from build123d import *

# Parameters (mm, degrees)
F1_DEPTH    = 30
F2_T1_DEPTH = 30
F2_T3_DEPTH = 35


# Not quite as in the source:
# - a fillet or chamfer that OpenCascade refuses, or shapes differently, is made with other operations: its cross-section is extruded or revolved along the edge and cut away or added
# - ends of sketch curves that miss each other by under 0.0002 mm in the source are joined


with BuildPart() as f1:
    # F0 (on Top) → F1 (new body)
    with BuildSketch(Plane.XY):
        with BuildLine():
            ThreePointArc((0.0108101467, 3.9999853926), (3.7311619501, 1.441676282), (2.6975556514, -2.9535052916))
            Line((2.6975556514, -2.9535052916), (3.5790398152, -3.7723300494))
            ThreePointArc((3.5790398152, -3.7723300494), (4.7376169007, -2.1435918693), (5.1962235425, -0.1981436252))
            ThreePointArc((5.1962235425, -0.1981436252), (5.1972192437, -0.0990548017), (5.2, 0))
            ThreePointArc((5.2, 0), (4.6973944029, 2.2303555374), (3.2867362218, 4.0295613915))
            Line((3.2867362218, 4.0295613915), (0.0108101467, 3.9999853926))
        make_face()
        with BuildLine():
            ThreePointArc((-2.6975556514, -2.9535052916), (-3.7272521414, 1.4517546193), (0.0108101467, 3.9999853926))
            Line((0.0108101467, 3.9999853926), (3.2867362218, 4.0295613915))
            ThreePointArc((3.2867362218, 4.0295613915), (1.7444599113, 4.8986589612), (0, 5.2))
            ThreePointArc((0, 5.2), (-4.8299128489, 1.9266400472), (-3.5790398152, -3.7723300494))
            Line((-3.5790398152, -3.7723300494), (-2.6975556514, -2.9535052916))
        make_face()
        with BuildLine():
            ThreePointArc((0, 5.2), (1.7444599113, 4.8986589612), (3.2867362218, 4.0295613915))
            Line((3.2867362218, 4.0295613915), (7.2283371129, 4.065071131))
            ThreePointArc((7.2283371129, 4.065071131), (8.8329374117, 4.9709020374), (10.646673336, 5.2959154939))
            Line((10.646673336, 5.2959154939), (0, 5.2))
        make_face()
        with BuildLine():
            ThreePointArc((5.2, 0), (5.1972192437, -0.0990548017), (5.1962235425, -0.1981436252))
            ThreePointArc((5.1962235425, -0.1981436252), (5.1990557999, -0.099089805), (5.2, 0))
        make_face()
        with BuildLine():
            ThreePointArc((5.2, 0), (5.1990557999, -0.099089805), (5.1962235425, -0.1981436252))
            ThreePointArc((5.1962235425, -0.1981436252), (5.5915030666, -2.2512643656), (6.7244861035, -4.0085065559))
            Line((6.7244861035, -4.0085065559), (7.5779271506, -3.1646460444))
            ThreePointArc((7.5779271506, -3.1646460444), (6.7375812297, 1.4751784497), (10.6574836162, 4.0959641875))
            Line((10.6574836162, 4.0959641875), (7.2283371129, 4.065071131))
            ThreePointArc((7.2283371129, 4.065071131), (5.7748395568, 2.2517463212), (5.2, 0))
        make_face()
        with BuildLine():
            ThreePointArc((10.646673336, 5.2959154939), (8.8329374117, 4.9709020374), (7.2283371129, 4.065071131))
            Line((7.2283371129, 4.065071131), (10.6574836162, 4.0959641875))
            Line((10.6574836162, 4.0959641875), (14.0866300839, 4.1268572436))
            ThreePointArc((14.0866300839, 4.1268572436), (12.4659704087, 5.0036318817), (10.646673336, 5.2959154939))
        make_face()
        with BuildLine():
            Line((16.1859897918, 5.345818995), (10.646673336, 5.2959154939))
            ThreePointArc((10.646673336, 5.2959154939), (12.4659704087, 5.0036318817), (14.0866300839, 4.1268572436))
            Line((14.0866300839, 4.1268572436), (17.6967392423, 4.1593805861))
            Line((17.6967392423, 4.1593805861), (17.6859289245, 5.3593318922))
            Line((17.6859289245, 5.3593318922), (16.1859897918, 5.345818995))
        make_face()
        with BuildLine():
            Line((14.0866300839, 4.1268572436), (10.6574836162, 4.0959641875))
            ThreePointArc((10.6574836162, 4.0959641875), (14.6395734892, 1.510772092), (13.8145139904, -3.1646460444))
            Line((13.8145139904, -3.1646460444), (14.6679550375, -4.0085065559))
            ThreePointArc((14.6679550375, -4.0085065559), (16.1822325131, 0.1881501089), (14.0866300839, 4.1268572436))
        make_face()
        Polygon((16.1634682964, 7.8457175493), (16.1859897918, 5.345818995), (17.6859289245, 5.3593318922), (17.6634074291, 7.8592304466), align=None)
        Polygon((-0.0225214954, 7.6998985544), (16.1634682964, 7.8457175493), (17.6634074291, 7.8592304466), (17.6498945318, 9.3591695792), (-0.0360343926, 9.199837687), (-4.7136558579, 9.1576971649), (-4.7001429606, 7.6577580323), align=None)
    extrude(amount=F1_DEPTH)

    # F2: fillet of radius 1 on 6 edges, made by hand

    # F2_s2 → F2_t1 (join)
    with BuildSketch(Plane.XY):
        with BuildLine():
            ThreePointArc((15.1635088747, 7.8367089512), (15.87322552, 7.5501976583), (16.1724768946, 6.8457581276))
            Line((16.1724768946, 6.8457581276), (16.1634682964, 7.8457175493))
            Line((16.1634682964, 7.8457175493), (15.1635088747, 7.8367089512))
        make_face()
        with BuildLine():
            ThreePointArc((16.1769811937, 6.3457784167), (15.8904699008, 5.6360617714), (15.1860303701, 5.3368103968))
            Line((15.1860303701, 5.3368103968), (16.1859897918, 5.345818995))
            Line((16.1859897918, 5.345818995), (16.1769811937, 6.3457784167))
        make_face()
    extrude(amount=F2_T1_DEPTH)

    # F2_s4 → F2_t3 (cut)
    with BuildSketch(Plane.XY.offset(-2.5)):
        with BuildLine():
            ThreePointArc((16.6967798205, 4.1503719879), (17.4012193512, 4.4496233625), (17.6877306441, 5.1593400078))
            Line((17.6877306441, 5.1593400078), (17.6967392423, 4.1593805861))
            Line((17.6967392423, 4.1593805861), (16.6967798205, 4.1503719879))
        make_face()
        with BuildLine():
            ThreePointArc((17.65890313, 8.3592101575), (17.3596517554, 9.0636496882), (16.6499351101, 9.3501609811))
            Line((16.6499351101, 9.3501609811), (17.6498945318, 9.3591695792))
            Line((17.6498945318, 9.3591695792), (17.65890313, 8.3592101575))
        make_face()
        with BuildLine():
            ThreePointArc((-3.7136964361, 9.1667057631), (-4.4181359668, 8.8674543885), (-4.7046472597, 8.1577377432))
            Line((-4.7046472597, 8.1577377432), (-4.7136558579, 9.1576971649))
            Line((-4.7136558579, 9.1576971649), (-3.7136964361, 9.1667057631))
        make_face()
        with BuildLine():
            ThreePointArc((-4.7091515588, 8.657717454), (-4.4099001842, 7.9532779233), (-3.7001835389, 7.6667666304))
            Line((-3.7001835389, 7.6667666304), (-4.7001429606, 7.6577580323))
            Line((-4.7001429606, 7.6577580323), (-4.7091515588, 8.657717454))
        make_face()
    extrude(amount=F2_T3_DEPTH, mode=Mode.SUBTRACT)


solid = f1.part
Verification items for the finished model (mm, model axes). A direction names the side the tool comes from. Coordinates: 2 decimals unless noted, no trailing zeros. Order: outer loops, then holes, each group sorted by start corner. A loop starts at its lowest first (then second) coordinate and runs counter-clockwise, first axis right, second up.
1. Sectioned sample at B-B, the plane y = -1.75. Record the cut outline in (x, z).
Results found:
outline: (-4.9, 0) - (-3.6, 0) - (-3.6, 30) - (-4.9, 30) - close; (3.6, 0) - (4.9, 0) - (4.9, 30) - (3.6, 30) - close; (5.42, 0) - (6.68, 0) - (6.68, 30) - (5.42, 30) - close; (14.71, 0) - (15.97, 0) - (15.97, 30) - (14.71, 30) - close
2. Scan lines: line 1 (X direction, y = -2.5, z = 12.75); line 2 (Y direction, x = 3.5, z = 6); line 3 (X direction, y = -1.25, z = 15). Record each from-to range of solid material in increasing order.
Results found:
line 1: x = -4.56 to -3.12, 3.12 to 4.56, 5.7 to 7.06, 14.33 to 15.69
line 2: y = -3.7 to -1.94, 1.94 to 3.85, 4.03 to 5.23, 7.73 to 9.23
line 3: x = -5.05 to -3.8, 3.8 to 5.05, 5.3 to 6.53, 14.87 to 16.1
3. Release check for a two-part mould opening along Y. For faces 1 (the face through (6.08, 4.25, 30)), 2 (the face through (5.8, 2.3, 14.8)), 3 (the face through (14.235, -3.581, 14.79)) record: +Y half, -Y half, draft (parallel to the pull), parting line (faces both ways), or undercut.
Results found:
face 1: draft
face 2: undercut
face 3: -Y half
4. Sectioned sample at C-C, the plane x = -1.5. Record the cut outline in (y, z), and give its area (3 significant figures).
Results found:
outline: (3.71, 0) - (4.98, 0) - (4.98, 30) - (3.71, 30) - close; (7.69, 0) - (9.19, 0) - (9.19, 30) - (7.69, 30) - close
area: 83.1 mm2
5. Sectioned sample at D-D, the plane y = 1.5. Record the cut outline in (x, z).
Results found:
outline: (-4.98, 0) - (-3.71, 0) - (-3.71, 30) - (-4.98, 30) - close; (3.71, 0) - (4.98, 0) - (4.98, 30) - (3.71, 30) - close; (5.47, 0) - (6.75, 0) - (6.75, 30) - (5.47, 30) - close; (14.64, 0) - (15.93, 0) - (15.93, 30) - (14.64, 30) - close
6. Sectioned sample at A-A, the plane z = 11.75. Record the cut outline in (x, y).
Results found:
outline: (-4.68, 8.41) arc R1 ccw to (-3.7, 7.67) - (15.16, 7.84) arc R1 cw to (16.17, 6.85) - (16.18, 6.35) arc R1 cw to (15.19, 5.34) - (0, 5.2) arc R5.2 ccw to (-3.58, -3.77) - (-2.7, -2.95) arc R4 cw (long way) to (2.7, -2.95) - (3.58, -3.77) arc R5.2 ccw to (5.2, -0.2) arc R5.5 ccw to (6.72, -4.01) - (7.58, -3.16) arc R4.3 cw (long way) to (13.81, -3.16) - (14.67, -4.01) arc R5.5 ccw to (14.09, 4.13) - (16.7, 4.15) arc R1 ccw to (17.69, 5.16) - (17.66, 8.36) arc R1 ccw to (16.65, 9.35) - (-3.71, 9.17) arc R1 ccw to start; hole (3.29, 4.03) arc R5.2 cw to (5.2, 0) arc R5.5 cw to (7.23, 4.07) - close
7. Go/stop test with flat-tipped pins: pin 1 Ø1 at (x, z) = (8, 20) entering from +Y; pin 2 Ø5 at (x, z) = (-2, 5.5) entering from +Y; pin 3 Ø1 at (y, z) = (6, 22.5) entering from -X. Record where each tip stops, or that it passes through.
Results found:
pin 1: stops at y = 9.28
pin 2: stops at y = 9.2
pin 3: stops at x = 15.72
8. Set-up check for faces 4 (the face through (15.865, 7.558, 14.79)), 5 (the face through (-4.317, 8.957, 14.79)), 6 (the face through (15.898, 5.644, 14.79)), 7 (the face through (6.08, 4.25, 0)), 8 (the face through (7.15, -3.59, 14.79)): record each of +Z, -Z, +X, -X, +Y, -Y from which the full face is reachable in a straight line by a thin tool's end or side.
Results found:
face 4: +Z, -Z
face 5: +Z, -Z, -X, +Y
face 6: +Z, -Z, -X
face 7: -Z, +X, -X, +Y, -Y
face 8: +Z, -Z, -Y
